Geometry check sheet. Reference: the model listing, model coordinates, mm. Face numbers are marked on the shaded views. A direction names the side the tool comes from. Round coordinates to 2 decimals unless told otherwise and drop trailing zeros. Write each loop counter-clockwise with the first axis right and the second up, starting at its lowest first coordinate (ties: lowest second). Pieces come first, ordered by that corner, then holes. Notation, with made-up numbers: M 81,35 L 128,35 A20 cw 128,71 Z; hole C -1.75,14 d4. An arc over 180 degrees is marked long. One line per item, written item: value. Start each with the question number.
1. Depth check by flat-ended pin: P1, Ø2, axis at x = -9.5, y = 95, coming from the +Z side; P2, Ø12, axis at x = 8, y = 122.5, coming from the -Z side; P3, Ø2, axis at x = -6.5, z = 11, coming from the -Y side. Enter the tip coordinate at first touch or a pass-through.
2. Section check C-C (x = 4.75). Record the boundary of the cut face in (y, z).
3. Scan lines: probe 1 along Y at (x, z) = (-10.75, -5.5); probe 2 along X at (y, z) = (-100.5, -7); probe 3 along X at (y, z) = (-38.5, -10.5). Record each from-to range of solid material in increasing order. Write a range as [from, to].
4. Access from +Z, -Z, +X, -X, +Y, -Y to the whole of each face (thin tool, end or side, straight path). Record for the marked faces 1, 2 and 3.
5. Section check D-D (y = -131.5). Record the boundary of the cut face in (x, z), and give its area (3 significant figures).
6. Section check B-B (y = 37). Record the boundary of the cut face in (x, z).
7. Section check A-A (z = 0). Record the boundary of the cut face in (x, y), and give its area (3 significant figures).
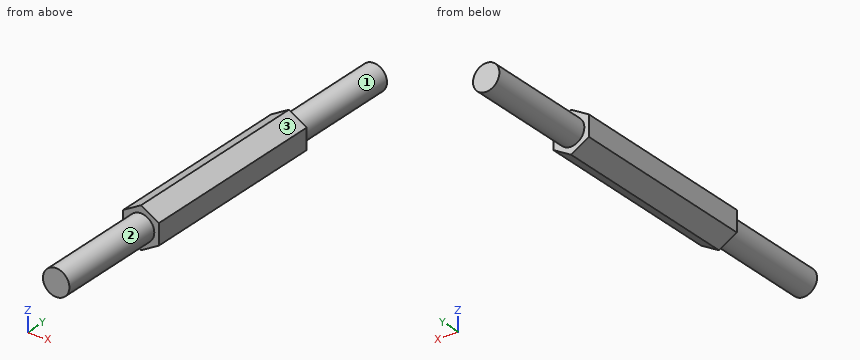
from build123d import *

# Parameters (mm, degrees)
F1_DEPTH = 74
F2_R     = 10
F3_DEPTH = 85


with BuildPart() as f1:
    # F0 (on Front) → F1 (new body)
    with BuildSketch(Plane.XZ):
        Polygon((13.5, -7.794229), (13.5, 7.794229), (0, 15.588457), (-13.5, 7.794229), (-13.5, -7.794229), (0, -15.588457), align=None)
    extrude(amount=F1_DEPTH)

    # F2 (on face) → F3 (join)
    with BuildSketch(Plane.XZ.offset(74)):
        Circle(F2_R)
    extrude(amount=F3_DEPTH)

    # F4: F1 across face


with BuildPart() as f1_1:
    add(f1.part)
    add(f1.part.mirror(Plane(origin=(0, 0, 0), x_dir=(1, 0, 0), z_dir=(0, 1, 0))))


solid = f1_1.part
Result sheet:
1. P1: stops at z = 5.27
1. P2: stops at z = -9.8
1. P3: stops at y = -74
2. outline: M -159,-8.8 L -74,-8.8 L -74,-12.85 L 74,-12.85 L 74,-8.8 L 159,-8.8 L 159,8.8 L 74,8.8 L 74,12.85 L -74,12.85 L -74,8.8 L -159,8.8 Z
3. probe 1: y = [-74, 74]
3. probe 2: x = [-7.14, 7.14]
3. probe 3: x = [-8.81, 8.81]
4. face 1: +Y
4. face 2: -Y
4. face 3: +Z, +X, +Y, -Y
5. outline: C 0,0 d20
5. area: 314 mm2
6. outline: M -13.5,-7.79 L 0,-15.59 L 13.5,-7.79 L 13.5,7.79 L 0,15.59 L -13.5,7.79 Z
7. outline: M -13.5,-74 L -10,-74 L -10,-159 L 10,-159 L 10,-74 L 13.5,-74 L 13.5,74 L 10,74 L 10,159 L -10,159 L -10,74 L -13.5,74 Z
7. area: 7,400 mm2
